Drawing for the job (mm, zero at the part's lowest x, y, z). Coordinates: 2 decimals unless noted, no trailing zeros. Loops run counter-clockwise (first coordinate to the right, second up) from the corner with the lowest first, then second, coordinate; pieces in that order, holes last. Notation, with made-up numbers: (45, 56.25) - (77, 56.25) arc R14 cw to (77, 78.25) - close; hole circle Ø11 at (45, 56.25). An arc over 180 degrees is marked (long way). Put each result on its own line as item: value.
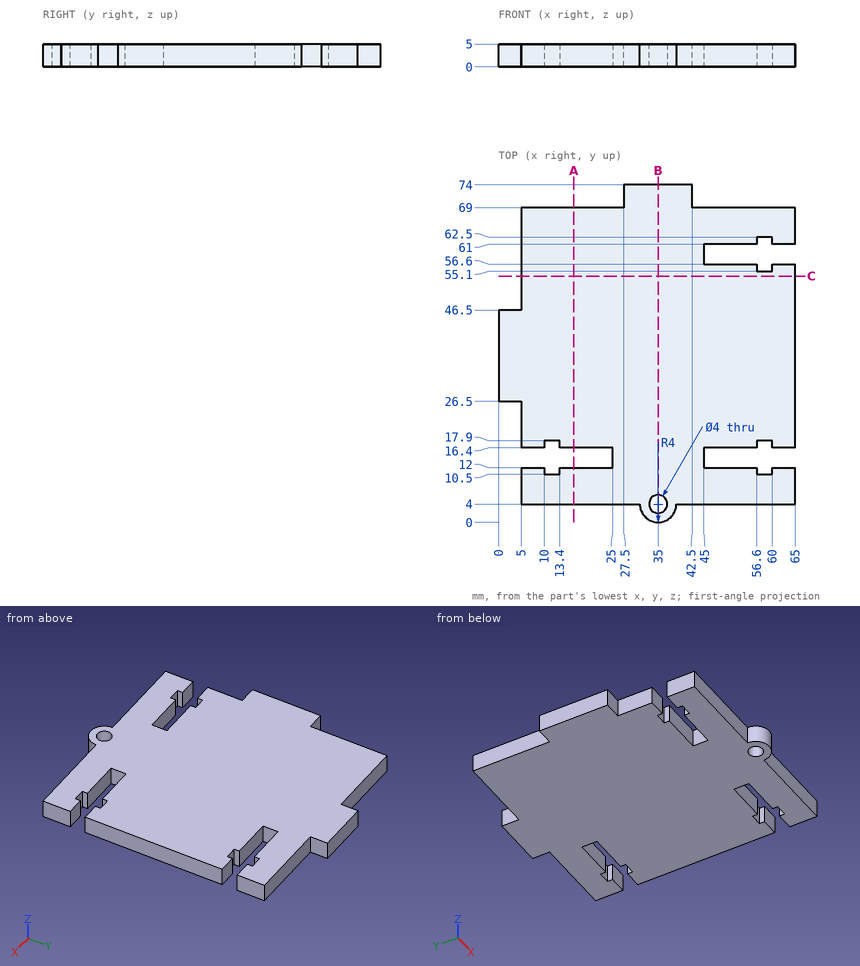
Q1. Pin check, flat tips, straight feed: pin 1 Ø2.5 at (x, z) = (63.5, 2) entering from +Y; pin 2 Ø3.5 at (x, y) = (35, 4) entering from +Z; pin 3 Ø1.5 at (y, z) = (72.5, 2.5) entering from -X; pin 4 Ø0.8 at (y, z) = (11.5, 3) entering from -X. Stop position of each tip, or through.
Determined:
pin 1: y = 69
pin 2: through
pin 3: x = 27.5
pin 4: x = 5
Q2. Slice it at B-B, the plane x = 35. Give the cut face in (y, z), then the cut area to 3 significant figures.
Determined:
outline: (0, 0) - (2, 0) - (2, 5) - (0, 5) - close; (6, 0) - (74, 0) - (74, 5) - (6, 5) - close
area: 350 mm2
Q3. Slice it at C-C, the plane y = 54. Give the cut face in (x, z), then the cut area to 3 significant figures.
Determined:
outline: (5, 0) - (65, 0) - (65, 5) - (5, 5) - close
area: 300 mm2
Q4. Slice it at A-A, the plane x = 16.5. Give the cut face in (y, z), then the cut area to 3 significant figures.
Determined:
outline: (4, 0) - (12, 0) - (12, 5) - (4, 5) - close; (16.4, 0) - (69, 0) - (69, 5) - (16.4, 5) - close
area: 303 mm2
Q5. Wall check: L1, parallel to Y at x = 47, z = 1.5; L2, parallel to X at y = 17.5, z = 2.8; L3, parallel to Y at x = 58, z = 3.3. Give the ranges that are in metal, low to high. Write a range as from..to.
Determined:
L1: 4..12, 16.4..56.6, 61..69
L2: 5..10, 13.4..56.6, 60..65
L3: 4..10.5, 17.9..55.1, 62.5..69
